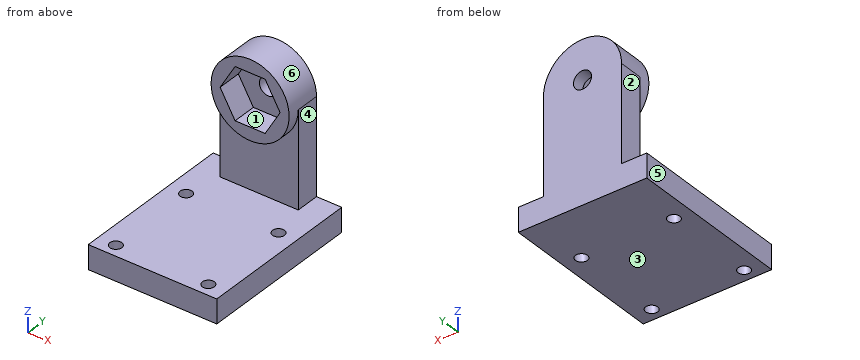
from build123d import *

# Parameters (mm, degrees)
SKETCH_2_R           = 6.5
EXTRUDE_1_DEPTH      = 6
CUT_EXTRUDE_1_DEPTH  = 4
SKETCH_3_R           = 1.5
CUT_EXTRUDE_2_DEPTH  = 4
EXTRUDE_START        = -4
EXTRUDE_2_DEPTH      = 4
EXTRUDE_6_DEPTH      = 4
SKETCH_17_R          = 1
CUT_EXTRUDE_11_DEPTH = 4


with BuildPart() as part:
    # 草图2 → 凸台-拉伸1 (new body)
    with BuildSketch(Plane(origin=(0, 0, 0), x_dir=(1, 0, 0), z_dir=(0, 1, 0))):
        with Locations(Location((0, 0, 0), (0, 0, 270))):
            Circle(SKETCH_2_R)
    extrude(amount=EXTRUDE_1_DEPTH)

    # 草图1 → 切除-拉伸1 (cut)
    with BuildSketch(Plane(origin=(0, 0, 0), x_dir=(1, 0, 0), z_dir=(0, 1, 0))):
        Polygon((5, 0), (2.5, 4.330127019), (-2.5, 4.330127019), (-5, 0), (-2.5, -4.330127019), (2.5, -4.330127019), align=None)
    extrude(amount=CUT_EXTRUDE_1_DEPTH, mode=Mode.SUBTRACT)

    # 草图3 → 切除-拉伸2 (cut)
    with BuildSketch(Plane(origin=(0, 6, 0), x_dir=(1, 0, 0), z_dir=(0, 1, 0))):
        with Locations(Location((0, 0, 0), (0, 0, 270))):
            Circle(SKETCH_3_R)
    extrude(amount=-CUT_EXTRUDE_2_DEPTH, mode=Mode.SUBTRACT)

    # 草图4 → 凸台-拉伸2 (add)
    with BuildSketch(Plane(origin=(0, 6, 0), x_dir=(1, 0, 0), z_dir=(0, 1, 0)).offset(EXTRUDE_START)):
        with BuildLine():
            Line((6.5, 0), (6.5, 20))
            Line((6.5, 20), (4, 20))
            Line((4, 20), (-4, 20))
            Line((-4, 20), (-6.5, 20))
            Line((-6.5, 20), (-6.5, 0))
            ThreePointArc((-6.5, 0), (0, 6.5), (6.5, 0))
        make_face()
    extrude(amount=EXTRUDE_2_DEPTH)

    # 草图6 → 凸台-拉伸6 (add)
    with BuildSketch(Plane(origin=(0, 0, -20), x_dir=(-1, 0, 0), z_dir=(0, 0, -1))):
        Polygon((10.7, -14.240758791), (10.7, 6), (-10.7, 6), (-10.7, -21.4), (10.7, -21.4), align=None)
    extrude(amount=-EXTRUDE_6_DEPTH)

    # 草图17 → 切除-拉伸11 (cut)
    with BuildSketch(Plane.XY.offset(-16)):
        with Locations((-7.7, -19.3)):
            Circle(SKETCH_17_R)
        with Locations((7.7, -19.3)):
            Circle(SKETCH_17_R)
        with Locations((7.7, -3.9)):
            Circle(SKETCH_17_R)
        with Locations((-7.7, -3.9)):
            Circle(SKETCH_17_R)
    extrude(amount=-CUT_EXTRUDE_11_DEPTH, mode=Mode.SUBTRACT)


solid = part.part
The model under review builds one solid part; all positions refer to its coordinate system, in mm. Face numbers are marked on the shaded views. A direction names the side the tool comes from. Give positions to 0.01 mm unless a question says otherwise; leave off trailing zeros. Order: outer loops, then holes, each group sorted by start corner. A loop starts at its lowest first (then second) coordinate and runs counter-clockwise, first axis right, second up. Notation, with made-up numbers: M 51,-38.75 L 61,-38.75 A27 ccw 61,-13.75 Z; hole C -4.75,-6.75 d10. An arc over 180 degrees is marked long. One line per question, with ' | ' between items. Start each with the question number.
1) Consider section D-D, the plane z = -5.25. Give the boundary of the cut face in (x, y), then the cut area to 3 significant figures.
2) Wall thickness on L1, parallel to Y at x = -7.7, z = -17.55; L2, parallel to Z at x = 2.25, y = 0.75; L3, parallel to X at y = 4.55, z = 0: over which ranges is each line inside the solid? List them lowest first. Write a range as from..to.
3) Consider section B-B, the plane y = -3.9. Give the boundary of the cut face in (x, z).
4) Consider section A-A, the plane x = -7.7. Give the boundary of the cut face in (y, z).
5) Mouldability with a two-part tool opening along Z and no side actions: class the marked faces 1, 2 and 3 as pulls with the +Z half, pulls with the -Z half, needs draft (parallel to the pull), parting line crosses it, or undercut.
6) Clearance check with flat-ended pins moving along their axes: P1, Ø4.5, axis at x = 0, z = -1.5, coming from the -Y side; P2, Ø4, axis at x = -6.5, y = 0, coming from the +Z side; P3, Ø3, axis at y = 3.5, z = -10, coming from the -X side; P4, Ø1.2, axis at x = 7.7, y = -19.3, coming from the +Z side. State where each tip first meets the part, or that it passes through.
7) Consider section C-C, the plane x = 0. Give the boundary of the cut face in (y, z).
8) For the marked faces 4, 5 and 6, list the 3-axis set-ups (+Z, -Z, +X, -X, +Y, -Y) from which the entire face can be reached by the end or side of a thin tool; tool diameter is ignored.
Found:
1) outline: M -6.5,2 L -3.83,2 L -3.83,0 L 3.83,0 L 3.83,2 L 6.5,2 L 6.5,6 L -6.5,6 Z | area: 67.3 mm²
2) L1: y = -21.4..-20.3, -18.3..-4.9, -2.9..6 | L2: z = -20..-16, -6.1..-4.33, 4.33..6.1 | L3: x = -6.5..-1.5, 1.5..6.5
3) outline: M -10.7,-20 L -8.7,-20 L -8.7,-16 L -10.7,-16 Z; M -6.7,-20 L 6.7,-20 L 6.7,-16 L -6.7,-16 Z; M 8.7,-20 L 10.7,-20 L 10.7,-16 L 8.7,-16 Z
4) outline: M -21.4,-20 L -20.3,-20 L -20.3,-16 L -21.4,-16 Z; M -18.3,-20 L -4.9,-20 L -4.9,-16 L -18.3,-16 Z; M -2.9,-20 L 6,-20 L 6,-16 L -2.9,-16 Z
5) face 1: undercut | face 2: needs draft | face 3: pulls with the -Z half
6) P1: stops at y = 4 | P2: stops at z = 4.69 | P3: stops at x = -6.5 | P4: passes through
7) outline: M -21.4,-20 L 6,-20 L 6,-1.5 L 4,-1.5 L 4,-4.33 L 0,-4.33 L 0,-6.5 L 2,-6.5 L 2,-16 L -21.4,-16 Z; M 0,4.33 L 4,4.33 L 4,1.5 L 6,1.5 L 6,6.5 L 0,6.5 Z
8) face 4: +Z, +X, +Y, -Y | face 5: +Z, -Z, -X, +Y, -Y | face 6: -Y
